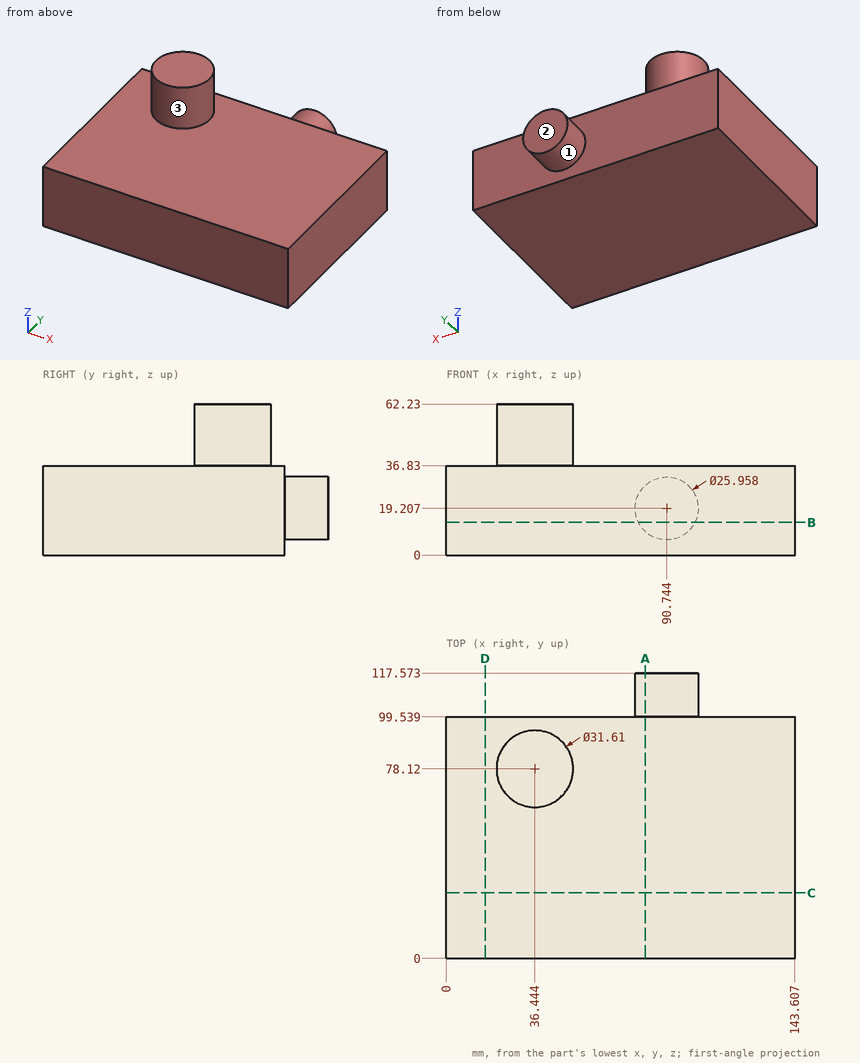
Design review of the part shown in the three views and the two pictorial views. Dimensions are in mm from the part's minimum x, y and z. A direction names the side the tool comes from. Round coordinates to 2 decimals unless told otherwise and drop trailing zeros. Loops run counter-clockwise (first coordinate to the right, second up) from the corner with the lowest first, then second, coordinate; pieces in that order, holes last.
Q1. Add section C-C on y = 27. Write out the cut boundary in (x, z), plus the area to 3 significant figures.
Result sheet:
outline: (0, 0) - (143.61, 0) - (143.61, 36.83) - (0, 36.83) - close
area: 5,290 mm2
Q2. Add section B-B on z = 13.5. Write out the cut boundary in (x, y).
Result sheet:
outline: (0, 0) - (143.61, 0) - (143.61, 99.54) - (102.4, 99.54) - (102.4, 117.57) - (79.09, 117.57) - (79.09, 99.54) - (0, 99.54) - close
Q3. To check wall thickness, follow line 1 along Y through (x, z) = (91.5, 5); line 2 along Z through (x, y) = (67, 46.5); line 3 along Y through (x, z) = (30.5, 53) (1 decimal). State the ranges of each line that lie inside material, in increasing order.
Result sheet:
line 1: y = 0 to 99.54
line 2: z = 0 to 36.83
line 3: y = 63.5 to 92.8
Q4. Add section A-A on x = 82. Write out the cut boundary in (y, z) (1 decimal), plus the area to 3 significant figures.
Result sheet:
outline: (0, 0) - (99.5, 0) - (99.5, 9.6) - (117.6, 9.6) - (117.6, 28.8) - (99.5, 28.8) - (99.5, 36.8) - (0, 36.8) - close
area: 4,010 mm2
Q5. Add section D-D on x = 16. Write out the cut boundary in (y, z), plus the area to 3 significant figures.
Result sheet:
outline: (0, 0) - (99.54, 0) - (99.54, 36.83) - (0, 36.83) - close
area: 3,670 mm2
Q6. Machinability: for the marked faces 1, 2 and 3, which of the approach directions +Z, -Z, +X, -X, +Y, -Y give a long, thin tool a straight path to every point of the face, cutting with its end or side? Answer none if there is none.
Result sheet:
face 1: +Y
face 2: +Z, -Z, +X, -X, +Y
face 3: +Z
Q7. Insertion check: pin 1 Ø1 at (x, z) = (34.5, 40.5) entering from +Y; pin 2 Ø8 at (x, y) = (84.5, 85) entering from +Z. Each pin has a flat end and moves straight along its axis. Give the tip position at first contact, or say it passes through.
Result sheet:
pin 1: stops at y = 93.86
pin 2: stops at z = 36.83
